from build123d import *

# Parameters (mm, degrees)
SKETCH1_W           = 6
SKETCH1_H           = 6
BOSS_EXTRUDE1_DEPTH = 1.5
FILLET1_R           = 0.3
SHELL1_START        = -2.7
SHELL1_OUTLINE_W    = 1.2
SHELL1_OUTLINE_H    = 5.4
SHELL1_DEPTH        = 5.4


# Read off the part's stored shape, not the designer's step: Shell1
with BuildPart() as part:
    # Sketch1 → Boss-Extrude1 (new body)
    with BuildSketch(Plane(origin=(0, 0, 0), x_dir=(1, 0, 0), z_dir=(0, 1, 0))):
        Rectangle(SKETCH1_W, SKETCH1_H)
    extrude(amount=BOSS_EXTRUDE1_DEPTH)

    # Fillet1
    fillet1_edges = [part.edges().sort_by_distance(p)[0] for p in [
        (-3, 1.5, 0),
        (0, 1.5, 3),
        (3, 1.5, 0),
        (3, 0.75, 3),
        (-3, 0.75, 3),
        (-3, 0.75, -3),
        (3, 0.75, -3),
        (0, 1.5, -3),
    ]]
    fillet(fillet1_edges, radius=FILLET1_R)

    # Shell1 outline → Shell1 (cut)
    with BuildSketch(Plane.YZ.offset(SHELL1_START)):
        with Locations((0.6, 0)):
            Rectangle(SHELL1_OUTLINE_W, SHELL1_OUTLINE_H)
    extrude(amount=SHELL1_DEPTH, mode=Mode.SUBTRACT)


solid = part.part
Can you work these out from the model? Positions are in its coordinate system, mm. A direction names the side the tool comes from. Coordinates: 2 decimals unless noted, no trailing zeros. Loops run counter-clockwise (first coordinate to the right, second up) from the corner with the lowest first, then second, coordinate; pieces in that order, holes last. Notation, with made-up numbers: (-32.5, -18) - (11.5, -18) arc R8 ccw to (11.5, -13) - close; hole circle Ø10 at (52.5, 82.25). An arc over 180 degrees is marked (long way). Answer as a JSON object with one key per item and string values. Group by question number.
Item 1: If we mould it in two halves opening along Z, with no side actions, what happens to faces 1 (the face through (0, 1, -3)), 2 (the face through (0, 1, 3)), 3 (the face through (-2.7, 1, 0)), 4 (the face through (3, 1, 0))? For each: released by +Z, released by -Z, zero draft, split by the parting line, or undercut.
Item 2: On a 3-axis mill with a long thin cutter (end or side, diameter ignored), from which of +Z, -Z, +X, -X, +Y, -Y can I reach the whole of each face in a straight line? I mean faces 5 (the face through (0, 1.5, 0)), 6 (the face through (0, 1, -2.7)). Say none if no direction works.
Item 3: If we section it at D-D (y = 1.35): List the corners of the cut face in (x, z) for me, plus the area to 3 significant figures.
Item 4: If we section it at A-A (y = 0.65): List the corners of the cut face in (x, z) for me.
Item 5: If we section it at C-C (x = -0.5): List the corners of the cut face in (y, z) for me, plus the area to 3 significant figures.
Item 6: If I drill on L1, parallel to Z at x = 1.95, y = 0.6; L2, parallel to Y at x = -1.25, z = 1.3, over which ranges is the centre line in solid material (lowest first)? Write a range as from..to.
Item 7: If we section it at B-B (z = 0.9): List the corners of the cut face in (x, y) for me, plus the area to 3 significant figures.
Item 8: For pin 1 (1.6 mm diameter, centred on x = 0.5, z = 1, fed in from -Y), with a flat end and sliding along its axis, tell me the tip position at first contact or that it passes through.
Returned:
{
 "1": {"face 1": "released by -Z", "face 2": "released by +Z", "face 3": "undercut", "face 4": "zero draft"},
 "2": {"face 5": "+Z, -Z, +X, -X, +Y", "face 6": "-Y"},
 "3": {"outline": "(-2.96, -2.7) arc R0.26 ccw to (-2.7, -2.96) - (2.7, -2.96) arc R0.26 ccw to (2.96, -2.7) - (2.96, 2.7) arc R0.26 ccw to (2.7, 2.96) - (-2.7, 2.96) arc R0.26 ccw to (-2.96, 2.7) - close", "area": "35.0 mm²"},
 "4": {"outline": "(-3, -2.7) arc R0.3 ccw to (-2.7, -3) - (2.7, -3) arc R0.3 ccw to (3, -2.7) - (3, 2.7) arc R0.3 ccw to (2.7, 3) - (-2.7, 3) arc R0.3 ccw to (-3, 2.7) - close; hole (-2.7, -2.7) - (2.7, -2.7) - (2.7, 2.7) - (-2.7, 2.7) - close"},
 "5": {"outline": "(0, -3) - (1.2, -3) arc R0.3 ccw to (1.5, -2.7) - (1.5, 2.7) arc R0.3 ccw to (1.2, 3) - (0, 3) - (0, 2.7) - (1.2, 2.7) - (1.2, -2.7) - (0, -2.7) - close", "area": "2.48 mm²"},
 "6": {"L1": "z = -3..-2.7, 2.7..3", "L2": "y = 1.2..1.5"},
 "7": {"outline": "(-3, 0) - (-2.7, 0) - (-2.7, 1.2) - (2.7, 1.2) - (2.7, 0) - (3, 0) - (3, 1.2) arc R0.3 ccw to (2.7, 1.5) - (-2.7, 1.5) arc R0.3 ccw to (-3, 1.2) - close", "area": "2.48 mm²"},
 "8": {"pin 1": "stops at y = 1.2"}
}
